from build123d import *

# Parameters (mm, degrees)
DODANIE_WYCI_GNI_CIE1_DEPTH = 580
KONWERTUJ_BRY_1_DEPTH       = 580
KONWERTUJ_BRY_1_2_DEPTH     = 580
OTW_R1_D                    = 4
LUSTRO2_COPY_1_D            = 4
OTW_R2_D                    = 4
SZKIC7_R                    = 2
WYTNIJ_WYCI_GNI_CIE1_DEPTH  = 584.86642308
LUSTRO5_COPY_1_SKETCH_R     = 2
LUSTRO5_COPY_1_DEPTH        = 584.86642308


# Read off the part's stored shape, not the designer's step: Konwertuj bryłę1
with BuildPart() as part:
    # Szkic2 → Dodanie-wyciągnięcie1 (new body)
    with BuildSketch(Plane.XY):
        Polygon((0, 0), (0, 30), (0, 60), (-3, 60), (-3, 45), (-30, 45), (-30, 30), (-30, 15), (-3, 15), (-3, 0), align=None)
    extrude(amount=DODANIE_WYCI_GNI_CIE1_DEPTH)

    # Konwertuj bryłę1 outline → Konwertuj bryłę1 (cut)
    with BuildSketch(Plane.XY):
        with BuildLine():
            Line((-30, 45), (-30, 41))
            ThreePointArc((-30, 41), (-28.828427125, 43.828427125), (-26, 45))
            Line((-26, 45), (-30, 45))
        make_face()
        with BuildLine():
            Line((-30, 15), (-26, 15))
            ThreePointArc((-26, 15), (-28.828427125, 16.171572875), (-30, 19))
            Line((-30, 19), (-30, 15))
        make_face()
        with BuildLine():
            Line((-26, 18), (-4, 18))
            ThreePointArc((-4, 18), (-1.171572875, 16.828427125), (0, 14))
            Line((0, 14), (0, 46))
            ThreePointArc((0, 46), (-1.171572875, 43.171572875), (-4, 42))
            Line((-4, 42), (-26, 42))
            ThreePointArc((-26, 42), (-26.707106781, 41.707106781), (-27, 41))
            Line((-27, 41), (-27, 19))
            ThreePointArc((-27, 19), (-26.707106781, 18.292893219), (-26, 18))
        make_face()
    extrude(amount=KONWERTUJ_BRY_1_DEPTH, mode=Mode.SUBTRACT)

    # Konwertuj bry_1 2 outline → Konwertuj bry_1 2 (add)
    with BuildSketch(Plane.XY):
        with BuildLine():
            ThreePointArc((-3, 46), (-3.292893219, 45.292893219), (-4, 45))
            Line((-4, 45), (-3, 45))
            Line((-3, 45), (-3, 46))
        make_face()
        with BuildLine():
            ThreePointArc((-4, 15), (-3.292893219, 14.707106781), (-3, 14))
            Line((-3, 14), (-3, 15))
            Line((-3, 15), (-4, 15))
        make_face()
    extrude(amount=KONWERTUJ_BRY_1_2_DEPTH)

    # Otwór1 (through all)
    with Locations(Plane.ZY.offset(3)):
        with Locations((573, 53), (565, 53)):
            otw_r1 = Hole(OTW_R1_D / 2)

    # Lustro1: Otwór1 across plane
    add(otw_r1.mirror(Plane(origin=(0, 30, 0), x_dir=(0, 0, 1), z_dir=(0, -1, 0))), mode=Mode.SUBTRACT)

    # Lustro2: Otwór1 across plane
    add(otw_r1.mirror(Plane.XY.offset(290)), mode=Mode.SUBTRACT)

    # Lustro2 copy 1 (through all)
    with Locations(Plane(origin=(-3, 60, 580), x_dir=(0, 0, -1), z_dir=(-1, 0, 0))):
        with Locations((573, 53), (565, 53)):
            Hole(LUSTRO2_COPY_1_D / 2)

    # Otwór2 (through all)
    with Locations(Plane.ZY.offset(3)):
        with Locations((290, 53)):
            otw_r2 = Hole(OTW_R2_D / 2)

    # Lustro3: Otwór2 across plane
    add(otw_r2.mirror(Plane(origin=(0, 30, 0), x_dir=(0, 0, 1), z_dir=(0, -1, 0))), mode=Mode.SUBTRACT)

    # Szkic7 → Wytnij-wyciągnięcie1 (cut, through all)
    with BuildSketch(Plane.ZY.offset(30)):
        with Locations(Location((4.25, 34.25, 0), (0, 0, 270))):
            Circle(SZKIC7_R)
    wytnij_wyci_gni_cie1 = extrude(amount=-WYTNIJ_WYCI_GNI_CIE1_DEPTH, mode=Mode.SUBTRACT)

    # Lustro4: Wytnij-wyciągnięcie1 across plane
    add(wytnij_wyci_gni_cie1.mirror(Plane.XY.offset(290)), mode=Mode.SUBTRACT)

    # Lustro5: Wytnij-wyciągnięcie1 across plane
    add(wytnij_wyci_gni_cie1.mirror(Plane(origin=(0, 30, 0), x_dir=(0, 0, 1), z_dir=(0, -1, 0))), mode=Mode.SUBTRACT)

    # Lustro5 copy 1 sketch → Lustro5 copy 1 (cut, through all)
    with BuildSketch(Plane(origin=(-30, 60, 580), x_dir=(0, 0, -1), z_dir=(-1, 0, 0))):
        with Locations(Location((4.25, 34.25, 0), (0, 0, 270))):
            Circle(LUSTRO5_COPY_1_SKETCH_R)
    extrude(amount=-LUSTRO5_COPY_1_DEPTH, mode=Mode.SUBTRACT)


solid = part.part
Work out the finished part from the listing and answer in its coordinate system (mm). A direction names the side the tool comes from. Give positions to 0.01 mm unless a question says otherwise; leave off trailing zeros. Order: outer loops, then holes, each group sorted by start corner. A loop starts at its lowest first (then second) coordinate and runs counter-clockwise, first axis right, second up. Notation, with made-up numbers: (85.5, 80) -> (89.5, 80) arc R5 ccw to (89.5, 86) -> close; hole circle Ø7 at (-36, 73). An arc over 180 degrees is marked (long way). Answer as a JSON object with one key per item and string values. Group by question number.
1. A tool of negligible diameter and unlimited length cuts with its end or side. For faces 1 (the flat face through (-3, 53, 286)), 2 (the flat face through (-15, 42, 286)), 3 (the flat face through (-15, 15, 286)), from which of +Z, -Z, +X, -X, +Y, -Y can it reach the whole face along a straight path? Write none if from no direction.
2. Section A-A on x = -10 is taken. Determine the outline of the cut face in (y, z).
3. Flat-ended cylindrical pins translate along their axes: pin 1 Ø6.5 at (x, z) = (-19.5, 245.5) entering from +Y; pin 2 Ø5 at (y, z) = (25.75, 575.75) entering from -X; pin 3 Ø4.5 at (y, z) = (34.25, 575.75) entering from +X; pin 4 Ø6 at (x, z) = (-23, 370) entering from -Y. Find the tip coordinate at first contact, or state that the pin passes through.
4. The mould has two halves that part along Y. Classify faces 4 (the flat face through (-30, 30, 286)), 5 (the flat face through (-15, 45, 286)), 6 (the flat face through (-27, 30, 286)): released by +Y, released by -Y, zero draft, split by the parting line, or undercut.
5. Consider line 1 along Y through (x, z) = (-1.65, 7); line 2 along Y through (x, z) = (-2.2, 573); line 3 along Y through (x, z) = (-11.5, 256). Determine where each line is inside the solid, lowest interval first. Write a range as [from, to].
Result sheet:
{
 "1": {"face 1": "+Z, -Z, -X, +Y", "face 2": "+Z, -Z, +X", "face 3": "+Z, -Z, -X, -Y"},
 "2": {"outline": "(15, 0) -> (18, 0) -> (18, 580) -> (15, 580) -> close; (42, 0) -> (45, 0) -> (45, 580) -> (42, 580) -> close"},
 "3": {"pin 1": "stops at y = 45", "pin 2": "stops at x = -30", "pin 3": "stops at x = -27", "pin 4": "stops at y = 15"},
 "4": {"face 4": "zero draft", "face 5": "released by +Y", "face 6": "undercut"},
 "5": {"line 1": "y = [0, 5], [9, 17.24], [42.76, 51], [55, 60]", "line 2": "y = [0, 5], [9, 17.57], [42.43, 51], [55, 60]", "line 3": "y = [15, 18], [42, 45]"}
}
